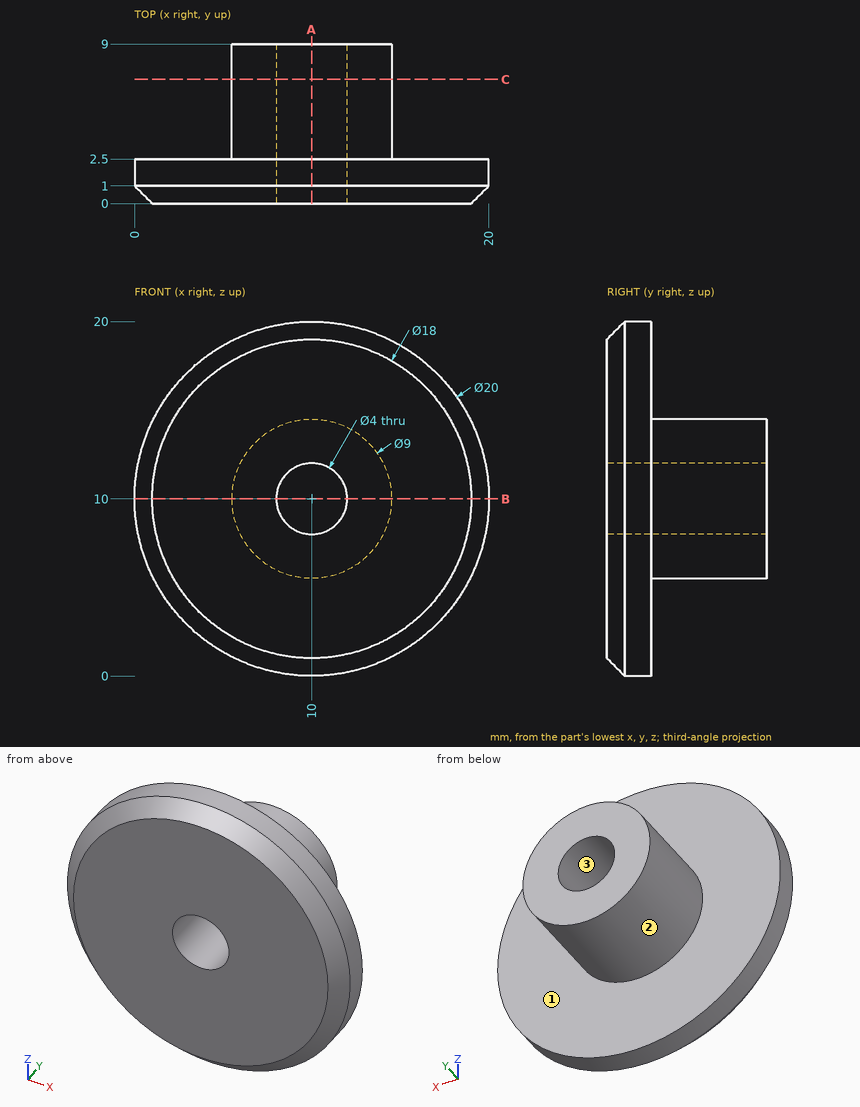
Geometry check sheet. Reference: drawing and pictorial views, mm from the part's lowest x, y, z. Coordinates: 2 decimals unless noted, no trailing zeros. Order: outer loops, then holes, each group sorted by start corner. A loop starts at its lowest first (then second) coordinate and runs counter-clockwise, first axis right, second up.
Item 1: Section check A-A, the plane x = 10. Enter the section's corners in (y, z), then the cut area to 3 significant figures.
Filled in:
outline: (0, 1) - (1, 0) - (2.5, 0) - (2.5, 5.5) - (9, 5.5) - (9, 8) - (0, 8) - close; (0, 12) - (9, 12) - (9, 14.5) - (2.5, 14.5) - (2.5, 20) - (1, 20) - (0, 19) - close
area: 71.5 mm2
Item 2: Release check for a two-part mould opening along Z. For the marked faces 1, 2 and 3 record: +Z half, -Z half, draft (parallel to the pull), parting line (faces both ways), or undercut.
Filled in:
face 1: draft
face 2: parting line
face 3: undercut
Item 3: Section check C-C, the plane y = 7. Enter the section's corners in (x, z).
Filled in:
outline: circle Ø9 at (10, 10); hole circle Ø4 at (10, 10)
Item 4: Material ranges on L1, parallel to Z at x = 10, y = 3.25; L2, parallel to Y at x = 8.75, z = 3; L3, parallel to Z at x = 11.5, y = 2.25, recorded low to high.
Filled in:
L1: z = 5.5 to 8, 12 to 14.5
L2: y = 0 to 2.5
L3: z = 0.11 to 8.68, 11.32 to 19.89
Item 5: Section check B-B, the plane z = 10. Enter the section's corners in (x, y), then the cut area to 3 significant figures.
Filled in:
outline: (0, 1) - (1, 0) - (8, 0) - (8, 9) - (5.5, 9) - (5.5, 2.5) - (0, 2.5) - close; (12, 0) - (19, 0) - (20, 1) - (20, 2.5) - (14.5, 2.5) - (14.5, 9) - (12, 9) - close
area: 71.5 mm2
Item 6: Depth check by flat-ended pin: pin 1 (3 mm diameter, centred on y = 6, z = 15.5, fed in from -X); pin 2 (2 mm diameter, centred on x = 7, z = 4, fed in from +Y); pin 3 (2 mm diameter, centred on y = 2, z = 6, fed in from +X). Enter the tip coordinate at first touch or a pass-through.
Filled in:
pin 1: stops at x = 7.94
pin 2: stops at y = 2.5
pin 3: stops at x = 19.54
